Check sheet for the modelled part. Datum: model origin and axes. Units: mm. Face numbers are marked on the shaded views. A direction names the side the tool comes from. Round coordinates to 2 decimals unless told otherwise and drop trailing zeros. Loops run counter-clockwise (first coordinate to the right, second up) from the corner with the lowest first, then second, coordinate; pieces in that order, holes last. Notation, with made-up numbers: (15, 52) -> (57, 52) arc R3 ccw to (57, 56) -> close; hole circle Ø11 at (8.25, 50.25). An arc over 180 degrees is marked (long way). Use one line per item in the form item = value. Start each with the question number.
(1) Material ranges on probe 1 along X at (y, z) = (3.5, 23.85); probe 2 along Y at (x, z) = (130.5, 24.25); probe 3 along Y at (x, z) = (64, 22.25), recorded low to high. Write a range as [from, to].
(2) Sectioned sample at A-A (y = 18.5). Record the cut outline in (x, z).
(3) Sectioned sample at C-C (x = 3). Record the cut outline in (y, z).
(4) Set-up check for the marked faces 1 and 2: record each of +Z, -Z, +X, -X, +Y, -Y from which the full face is reachable in a straight line by a thin tool's end or side.
(5) Sectioned sample at B-B (z = 10.25). Record the cut outline in (x, y).
(6) Draft check along X on the marked faces 3, 4, 5 and 6. Enter one of: released by +X, released by -X, zero draft, split by the parting line, or undercut.
(7) Sectioned sample at D-D (y = 3.5). Record the cut outline in (x, z), and give its area (3 significant figures).
(8) Go/stop test with flat-tipped pins: pin 1 (0.9 mm diameter, centred on x = 3, y = 70, fed in from +Z); pin 2 (6 mm diameter, centred on x = 116, y = 43.5, fed in from +Z); pin 3 (2 mm diameter, centred on x = 128, y = 62.5, fed in from +Z). Record where each tip stops, or that it passes through.
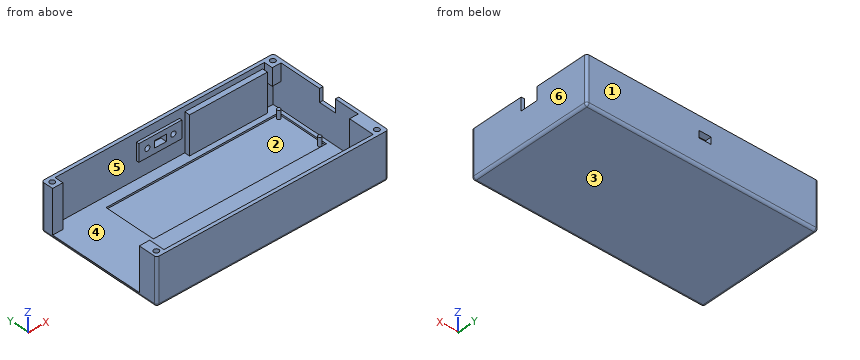
from build123d import *

# Parameters (mm, degrees)
BOX_W             = 134
BOX_H             = 73
BOX_DEPTH         = 27
BOX001_W          = 126
BOX001_H          = 69
BOX001_DEPTH      = 25
BOX002_W          = 10
BOX002_H          = 55
BOX002_DEPTH      = 25
BOX003_W          = 100
BOX003_H          = 30
BOX003_DEPTH      = 1
CYLINDER_R        = 1
CYLINDER_DEPTH    = 5
CYLINDER001_R     = 1
CYLINDER001_DEPTH = 5
BOX004_W          = 25
BOX004_H          = 1.5
BOX004_DEPTH      = 10
BOX005_W          = 7
BOX005_H          = 4
BOX005_DEPTH      = 7
CYLINDER002_R     = 1.5
CYLINDER002_DEPTH = 2.5
CYLINDER003_R     = 1.5
CYLINDER003_DEPTH = 2.5
BOX006_W          = 45
BOX006_H          = 22
BOX006_DEPTH      = 3
BOX007_W          = 7.5
BOX007_H          = 10
BOX007_DEPTH      = 2
BOX008_W          = 15
BOX008_H          = 5
BOX008_DEPTH      = 25
BOX009_W          = 5
BOX009_H          = 5
BOX009_DEPTH      = 10
CYLINDER004_R     = 1.5
CYLINDER004_DEPTH = 5
CYLINDER005_R     = 1.5
CYLINDER005_DEPTH = 5
CYLINDER006_R     = 1.5
CYLINDER006_DEPTH = 5
CYLINDER007_R     = 1.5
CYLINDER007_DEPTH = 5
FILLET_R          = 1.5
FILLET001_R       = 1.5
FILLET002_R       = 1.5
FILLET003_R       = 1.5


with BuildPart() as part:
    # Box → Box (join)
    with BuildSketch(Plane.XY):
        with Locations((67, 36.5)):
            Rectangle(BOX_W, BOX_H)
    extrude(amount=BOX_DEPTH)

    # Box001 → Box001 (cut)
    with BuildSketch(Plane(origin=(6, 2, 2), x_dir=(1, 0, 0), z_dir=(0, 0, 1))):
        with Locations((63, 34.5)):
            Rectangle(BOX001_W, BOX001_H)
    extrude(amount=BOX001_DEPTH, mode=Mode.SUBTRACT)

    # Box002 → Box002 (cut)
    with BuildSketch(Plane(origin=(-2, 11, 2), x_dir=(1, 0, 0), z_dir=(0, 0, 1))):
        with Locations((5, 27.5)):
            Rectangle(BOX002_W, BOX002_H)
    extrude(amount=BOX002_DEPTH, mode=Mode.SUBTRACT)

    # Box003 → Box003 (cut)
    with BuildSketch(Plane(origin=(30, 35, 1), x_dir=(1, 0, 0), z_dir=(0, 0, 1))):
        with Locations((50, 15)):
            Rectangle(BOX003_W, BOX003_H)
    extrude(amount=BOX003_DEPTH, mode=Mode.SUBTRACT)

    # Cylinder → Cylinder (join)
    with BuildSketch(Plane(origin=(128, 37, 1), x_dir=(1, 0, 0), z_dir=(0, 0, 1))):
        Circle(CYLINDER_R)
    extrude(amount=CYLINDER_DEPTH)

    # Cylinder001 → Cylinder001 (join)
    with BuildSketch(Plane(origin=(128, 63, 1), x_dir=(1, 0, 0), z_dir=(0, 0, 1))):
        Circle(CYLINDER001_R)
    extrude(amount=CYLINDER001_DEPTH)

    # Box004 → Box004 (join)
    with BuildSketch(Plane(origin=(53, 69.5, 12), x_dir=(1, 0, 0), z_dir=(0, 0, 1))):
        with Locations((12.5, 0.75)):
            Rectangle(BOX004_W, BOX004_H)
    extrude(amount=BOX004_DEPTH)

    # Box005 → Box005 (cut)
    with BuildSketch(Plane(origin=(62, 74.5, 15), x_dir=(1, 0, 0), z_dir=(0, -1, 0))):
        with Locations((3.5, 2)):
            Rectangle(BOX005_W, BOX005_H)
    extrude(amount=BOX005_DEPTH, mode=Mode.SUBTRACT)

    # Cylinder002 → Cylinder002 (cut)
    with BuildSketch(Plane(origin=(58, 72, 17), x_dir=(1, 0, 0), z_dir=(0, -1, 0))):
        Circle(CYLINDER002_R)
    extrude(amount=CYLINDER002_DEPTH, mode=Mode.SUBTRACT)

    # Cylinder003 → Cylinder003 (cut)
    with BuildSketch(Plane(origin=(73, 72, 17), x_dir=(1, 0, 0), z_dir=(0, -1, 0))):
        Circle(CYLINDER003_R)
    extrude(amount=CYLINDER003_DEPTH, mode=Mode.SUBTRACT)

    # Box006 → Box006 (join)
    with BuildSketch(Plane(origin=(81, 71, 2), x_dir=(1, 0, 0), z_dir=(0, -1, 0))):
        with Locations((22.5, 11)):
            Rectangle(BOX006_W, BOX006_H)
    extrude(amount=BOX006_DEPTH)

    # Box007 → Box007 (cut)
    with BuildSketch(Plane(origin=(134, 41.5, 27), x_dir=(0, 0, -1), z_dir=(-1, 0, 0))):
        with Locations((3.75, 5)):
            Rectangle(BOX007_W, BOX007_H)
    extrude(amount=BOX007_DEPTH, mode=Mode.SUBTRACT)

    # Box008 → Box008 (join)
    with BuildSketch(Plane(origin=(132, 2, 2), x_dir=(0, 1, 0), z_dir=(0, 0, 1))):
        with Locations((7.5, 2.5)):
            Rectangle(BOX008_W, BOX008_H)
    extrude(amount=BOX008_DEPTH)

    # Box009 → Box009 (join)
    with BuildSketch(Plane(origin=(132, 66, 17), x_dir=(0, 1, 0), z_dir=(0, 0, 1))):
        with Locations((2.5, 2.5)):
            Rectangle(BOX009_W, BOX009_H)
    extrude(amount=BOX009_DEPTH)

    # Cylinder004 → Cylinder004 (cut)
    with BuildSketch(Plane(origin=(130.5, 69.5, 22), x_dir=(0, 1, 0), z_dir=(0, 0, 1))):
        Circle(CYLINDER004_R)
    extrude(amount=CYLINDER004_DEPTH, mode=Mode.SUBTRACT)

    # Cylinder005 → Cylinder005 (cut)
    with BuildSketch(Plane(origin=(130.5, 3.5, 22), x_dir=(0, 1, 0), z_dir=(0, 0, 1))):
        Circle(CYLINDER005_R)
    extrude(amount=CYLINDER005_DEPTH, mode=Mode.SUBTRACT)

    # Cylinder006 → Cylinder006 (cut)
    with BuildSketch(Plane(origin=(3, 3.5, 22), x_dir=(0, 1, 0), z_dir=(0, 0, 1))):
        Circle(CYLINDER006_R)
    extrude(amount=CYLINDER006_DEPTH, mode=Mode.SUBTRACT)

    # Cylinder007 → Cylinder007 (cut)
    with BuildSketch(Plane(origin=(3, 69.5, 22), x_dir=(0, 1, 0), z_dir=(0, 0, 1))):
        Circle(CYLINDER007_R)
    extrude(amount=CYLINDER007_DEPTH, mode=Mode.SUBTRACT)

    # Fillet
    fillet_edges = [part.edges().sort_by_distance(p)[0] for p in [
        (134, 0, 13.5),
    ]]
    fillet(fillet_edges, radius=FILLET_R)

    # Fillet001
    fillet001_edges = [part.edges().sort_by_distance(p)[0] for p in [
        (134, 73, 13.5),
    ]]
    fillet(fillet001_edges, radius=FILLET001_R)

    # Fillet002
    fillet002_edges = [part.edges().sort_by_distance(p)[0] for p in [
        (134, 36.5, 0),
    ]]
    fillet(fillet002_edges, radius=FILLET002_R)

    # Fillet003
    fillet003_edges = [part.edges().sort_by_distance(p)[0] for p in [
        (0, 73, 14.25),
        (0, 36.5, 0),
        (0, 0, 14.25),
    ]]
    fillet(fillet003_edges, radius=FILLET003_R)


solid = part.part
Checks:
q1.probe_1 = [0, 1.5], [4.5, 6], [127, 129], [132, 134]
q1.probe_2 = [0, 2], [5, 17], [66, 68], [71, 73]
q1.probe_3 = [0, 2], [71, 73]
q2.outline = (0, 1.5) arc R1.5 ccw to (1.5, 0) -> (132.5, 0) arc R1.5 ccw to (134, 1.5) -> (134, 27) -> (132, 27) -> (132, 2) -> (0, 2) -> close
q3.outline = (0, 1.5) arc R1.5 ccw to (1.5, 0) -> (71.5, 0) arc R1.5 ccw to (73, 1.5) -> (73, 27) -> (71, 27) -> (71, 22) -> (68, 22) -> (68, 27) -> (66, 27) -> (66, 2) -> (11, 2) -> (11, 27) -> (5, 27) -> (5, 22) -> (2, 22) -> (2, 27) -> (0, 27) -> close
q4.face_1 = +Z, -Z, +X, -X, +Y
q4.face_2 = +Z
q5.outline = (0, 1.5) arc R1.5 ccw to (1.5, 0) -> (132.5, 0) arc R1.5 ccw to (134, 1.5) -> (134, 71.5) arc R1.5 ccw to (132.5, 73) -> (1.5, 73) arc R1.5 ccw to (0, 71.5) -> (0, 66) -> (6, 66) -> (6, 71) -> (81, 71) -> (81, 68) -> (126, 68) -> (126, 71) -> (132, 71) -> (132, 17) -> (127, 17) -> (127, 2) -> (6, 2) -> (6, 11) -> (0, 11) -> close
q6.face_3 = zero draft
q6.face_4 = undercut
q6.face_5 = undercut
q6.face_6 = released by +X
q7.outline = (0, 1.5) arc R1.5 ccw to (1.5, 0) -> (132.5, 0) arc R1.5 ccw to (134, 1.5) -> (134, 27) -> (132, 27) -> (132, 22) -> (129, 22) -> (129, 27) -> (127, 27) -> (127, 2) -> (6, 2) -> (6, 27) -> (4.5, 27) -> (4.5, 22) -> (1.5, 22) -> (1.5, 27) -> (0, 27) -> close
q7.area = 562 mm2
q8.pin_1 = 22
q8.pin_2 = 1
q8.pin_3 = 6
